Could you check a few things on this drawing? It's one solid part, dimensions in mm from its lowest x, y, z. A direction names the side the tool comes from. Give positions to 0.01 mm unless a question says otherwise; leave off trailing zeros. Loops run counter-clockwise (first coordinate to the right, second up) from the corner with the lowest first, then second, coordinate; pieces in that order, holes last. Notation, with made-up numbers: (-0.75, 73.25) - (15.25, 73.25) arc R24 cw to (15.25, 91.25) - close; hole circle Ø10 at (58, -27.5). An arc over 180 degrees is marked (long way). Return JSON: item names as keys, results as strings. Group by question number.
(1) I need wall thicknesses on probe 1 along Z at (x, y) = (3.5, 2.15); probe 2 along X at (y, z) = (0.85, 10); probe 3 along X at (y, z) = (13.25, 57.5). Which ranges of each line are inside material? Lowest first, please. Write a range as [from, to].
(2) For P1, Ø2, axis at x = 4, z = 69, coming from the +Y side; P2, Ø2.5, axis at x = 13, y = 7.5, coming from the +Z side; P3, Ø6, axis at y = 12, z = 26.5, coming from the -X side, each with a flat end and sliding along its axis, tell me the tip position at first contact or that it passes through.
(3) On a 3-axis mill with a long thin cutter (end or side, diameter ignored), from which of +Z, -Z, +X, -X, +Y, -Y can I reach the whole of each face in a straight line? I mean the marked faces 1, 2 and 3. Say none if no direction works.
(4) If we section it at C-C (y = 7): Please give me the cut outline in (x, z), then the cut area to 3 significant figures.
(5) If we section it at A-A (x = 3.5): Please give me the cut outline in (y, z).
(6) If we section it at D-D (x = 11): Please give me the cut outline in (y, z), then the cut area to 3 significant figures.
(7) If we section it at B-B (z = 10): Please give me the cut outline in (x, y).
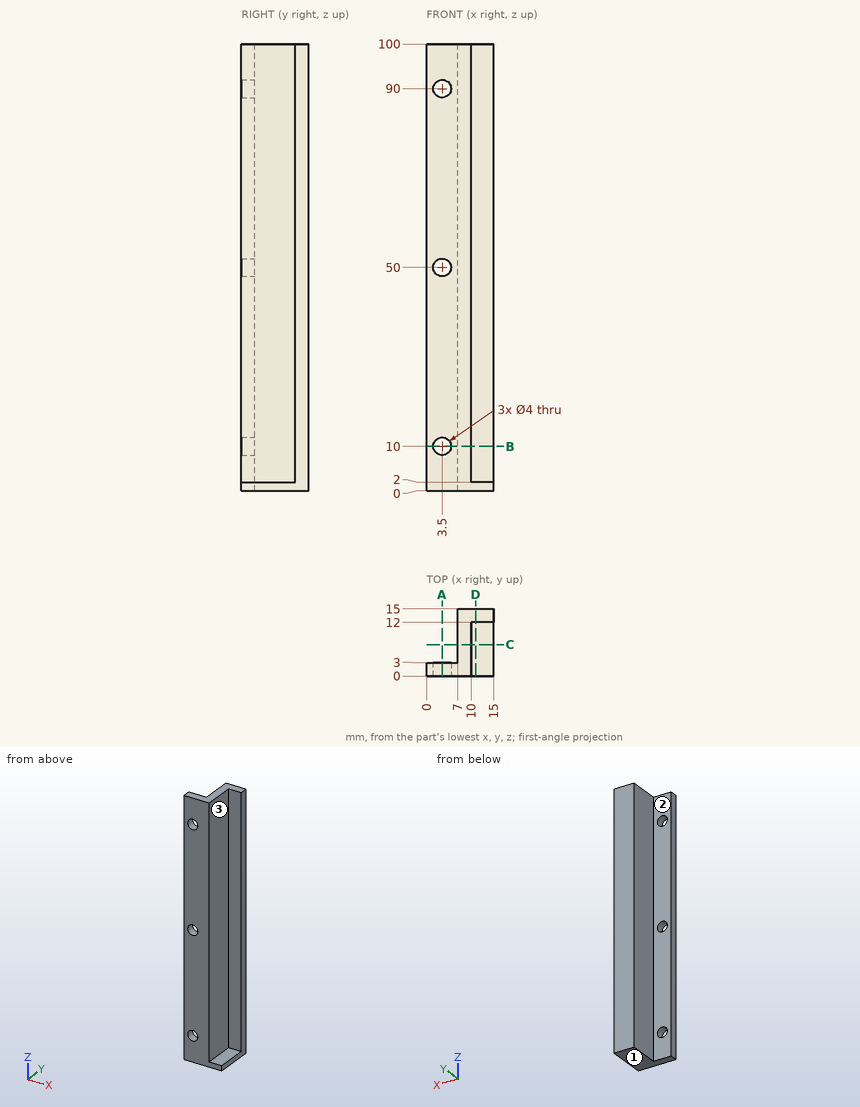
Values:
{
 "1": {"probe 1": "[0, 8], [12, 48], [52, 88], [92, 100]", "probe 2": "[0, 1.5], [5.5, 10]", "probe 3": "[7, 15]"},
 "2": {"P1": "y = 3", "P2": "z = 2", "P3": "x = 7"},
 "3": {"face 1": "-Z, +X, -X, +Y, -Y", "face 2": "+Z, -Z, -X, +Y", "face 3": "+Z, +X, -Y"},
 "4": {"outline": "(7, 0) - (15, 0) - (15, 2) - (10, 2) - (10, 100) - (7, 100) - close", "area": "310 mm2"},
 "5": {"outline": "(0, 0) - (3, 0) - (3, 8) - (0, 8) - close; (0, 12) - (3, 12) - (3, 48) - (0, 48) - close; (0, 52) - (3, 52) - (3, 88) - (0, 88) - close; (0, 92) - (3, 92) - (3, 100) - (0, 100) - close"},
 "6": {"outline": "(0, 0) - (15, 0) - (15, 100) - (12, 100) - (12, 2) - (0, 2) - close", "area": "324 mm2"},
 "7": {"outline": "(0, 0) - (1.5, 0) - (1.5, 3) - (0, 3) - close; (5.5, 0) - (10, 0) - (10, 12) - (15, 12) - (15, 15) - (7, 15) - (7, 3) - (5.5, 3) - close"}
}
